Read the model definition and answer for the solid it produces. Units are mm, in the model's axes. Give positions to 0.01 mm unless a question says otherwise; leave off trailing zeros. Write each loop counter-clockwise with the first axis right and the second up, starting at its lowest first coordinate (ties: lowest second). Pieces come first, ordered by that corner, then holes. Notation, with made-up numbers: (9.25, 31.25) -> (39.25, 31.25) arc R16 cw to (39.25, 38.25) -> close; hole circle Ø11 at (-22, -3). An arc over 180 degrees is marked (long way). Write item = value, one per line.
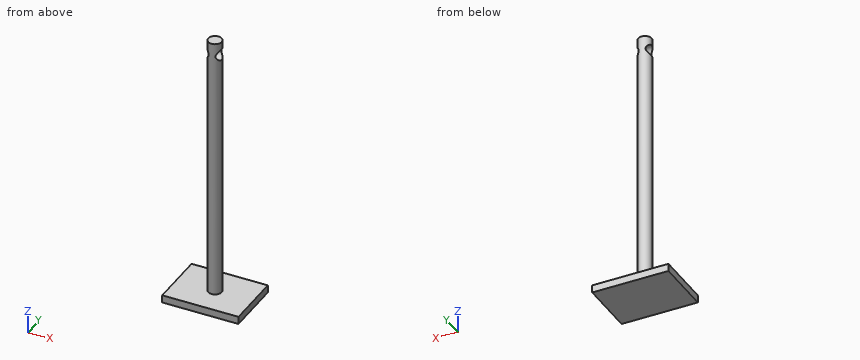
from build123d import *

# Parameters (mm, degrees)
F0_W     = 50.8
F0_H     = 5.08
F1_DEPTH = 38.1
F2_R     = 4.445
F3_DEPTH = 177.8
F4_R     = 3.81
F5_DEPTH = 50.673


with BuildPart() as f1:
    # F0 (on Front) → F1 (new body)
    with BuildSketch(Plane.XZ):
        with Locations((25.4, 2.54)):
            Rectangle(F0_W, F0_H)
    extrude(amount=F1_DEPTH)

    # F2 (on face) → F3 (join)
    with BuildSketch(Plane.XY.offset(5.08)):
        with Locations((25.4, -19.05)):
            Circle(F2_R)
    extrude(amount=F3_DEPTH)

    # F4 (on Right) → F5 (cut)
    with BuildSketch(Plane.YZ):
        with Locations((-19.05, 173.99)):
            Circle(F4_R)
    extrude(amount=F5_DEPTH, mode=Mode.SUBTRACT)


solid = f1.part
(1) The part is cut by section C-C on z = 173.99. Determine the outline of the cut face in (x, y) (3 decimals), plus the area to 3 significant figures.
Checks:
outline = (23.11, -22.86) arc R4.445 ccw to (27.69, -22.86) -> close; (23.11, -15.24) -> (27.69, -15.24) arc R4.445 ccw to start
area = 3.94 mm²
(2) The part is cut by section D-D on y = -33.5. Determine the outline of the cut face in (x, z), plus the area to 3 significant figures.
Checks:
outline = (0, 0) -> (50.8, 0) -> (50.8, 5.08) -> (0, 5.08) -> close
area = 258 mm²
(3) Consider L1, parallel to Z at x = 23.25, y = -19.05; L2, parallel to Y at x = 25.75, z = 173.99; L3, parallel to Z at x = 46, y = -15.5. Determine where each line is inside the solid, lowest interval first.
Checks:
L1 = 0 to 170.18, 177.8 to 182.88
L2 = -23.48 to -22.86, -15.24 to -14.62
L3 = 0 to 5.08
(4) The part is cut by section A-A on x = 25.4. Determine the outline of the cut face in (y, z) (3 decimals).
Checks:
outline = (-38.1, 0) -> (0, 0) -> (0, 5.08) -> (-14.605, 5.08) -> (-14.605, 182.88) -> (-23.495, 182.88) -> (-23.495, 5.08) -> (-38.1, 5.08) -> close; hole circle Ø7.62 at (-19.05, 173.99)
(5) The part is cut by section B-B on y = -19.05. Determine the outline of the cut face in (x, z) (3 decimals).
Checks:
outline = (0, 0) -> (50.8, 0) -> (50.8, 5.08) -> (29.845, 5.08) -> (29.845, 170.18) -> (20.955, 170.18) -> (20.955, 5.08) -> (0, 5.08) -> close; (20.955, 177.8) -> (29.845, 177.8) -> (29.845, 182.88) -> (20.955, 182.88) -> close
(6) Given P1, Ø1.5, axis at y = -15, z = 45.5, coming from the +X side; P2, Ø8, axis at x = 6.5, y = -22.5, coming from the +Z side; P3, Ø10, axis at x = 20.5, z = 129.5, coming from the -Y side (3 decimals), each flat-ended and moving along its own axis, determine where each tip first touches the part or whether it passes through.
Checks:
P1 = 28.38
P2 = 5.08
P3 = -23.495
